Design review of the part built by this model. Coordinates are the model's own, in mm. A direction names the side the tool comes from. Give positions to 0.01 mm unless a question says otherwise; leave off trailing zeros. Write each loop counter-clockwise with the first axis right and the second up, starting at its lowest first coordinate (ties: lowest second). Pieces come first, ordered by that corner, then holes. Notation, with made-up numbers: M 24,74.5 L 33,74.5 A13 cw 33,83.5 Z; hole C 80.25,-3 d1. An arc over 180 degrees is marked long. Write each question's results on one line, items separated by ' | '. Start each with the question number.
Autodesk Fusion 360 part; units mm, degrees
sketch "Sketch1" plane through (0, 0, 0) normal (0, 0, 1) x (1, 0, 0)
  circle A0 centre (0, 0) radius 22.75
  circle A1 centre (0, 0) radius 24.25
  dimension "d1" = 45.5
  dimension "d2" = 48.5
extrude "Extrude1" add sketch "Sketch1" along normal blind 33
sketch "Sketch2" plane through (0, 0, 0) normal (0, 1, 0) x (1, 0, 0)
  line L0 (-24.25, 0) -> (24.25, 0)
  line L1 (4.75, -6.25) -> (-4.75, -6.25)
  line L2 (-4.75, -6.25) -> (-4.75, -2.75)
  line L3 (-4.75, -2.75) -> (4.75, -2.75)
  line L4 (4.75, -2.75) -> (4.75, -6.25)
  line L5 (4.75, -6.25) -> (-4.75, -2.75) construction
  line L6 (-4.75, -6.25) -> (4.75, -2.75) construction
  point P0 (0, -4.5)
  dimension "d9" = 9.5
  dimension "d10" = 3.5
  dimension "d11" = 2.75
extrude "Extrude2" cut sketch "Sketch2" along normal mid plane 66
sketch "Sketch3" plane through (0, 0, 33) normal (0, 0, 1) x (-1, 0, 0)
  circle A0 centre (0, 0) radius 22.75
  circle A1 centre (0, 0) radius 24.25
  circle A2 centre (0, 0) radius 25
  circle A3 centre (0, 0) radius 22.75
extrude "Extrude3" add sketch "Sketch3" along normal blind 3 contours A1 | A2
sketch "Sketch4" plane through (0, 0, 36) normal (0, 0, 1) x (-1, 0, 0)
  circle A0 centre (0, 0) radius 22.75
  circle A1 centre (0, 0) radius 25
  circle A2 centre (0, 0) radius 23.25
  circle A3 centre (0, 0) radius 22
  dimension "d18" = 46.5
  dimension "d19" = 44
ref_plane "WorkPlane2" through (0, 0, 43) normal (0, 0, 1) x (-1, 0, 0)
sketch "Sketch6" plane through (0, 0, 43) normal (0, 0, 1) x (1, 0, 0)
  circle A0 centre (0, 0) radius 22
  circle A1 centre (0, 0) radius 23.25
  dimension "d26" = 44
  dimension "d27" = 46.5
extrude "Extrude4" add sketch "Sketch6" against normal blind 7
ref_plane "WorkPlane1" through (0, 0, 56) normal (0, 0, 1) x (-1, 0, 0)
sketch "Sketch5" plane through (0, 0, 56) normal (0, 0, 1) x (1, 0, 0)
  circle A0 centre (0, 0) radius 22.75
  circle A1 centre (0, 0) radius 21.25
  dimension "d21" = 45.5
  dimension "d22" = 42.5
loft "Loft1" add profiles "Sketch6", "Sketch5" section 1 section 2
loft "Loft2" cut profiles "Sketch5", "Sketch6" section 1 contours A1 section 2 contours A0
chamfer "Chamfer1" distance 1.75 angle 45 1 edges at (-21.6766, 8.4076, 36)
chamfer "Chamfer3" distance 0.75 angle 45 1 edges at (21.2104, -8.2268, 36)
chamfer "Chamfer4" distance 0.75 angle 45 1 edges at (-22.6089, -8.7692, 33)
fillet "Fillet1" radius 1.75 8 edges at (-4.75, -23.0144, 6.25) (-4.75, -23.0144, 2.75) (4.75, -23.0144, 6.25) (4.75, -23.0144, 2.75) (4.75, 23.0144, 2.75) (4.75, 23.0144, 6.25) (-4.75, 23.0144, 6.25) (-4.75, 23.0144, 2.75)
Q1. The part is to be moulded in two halves that separate along Y. For faces 4 (the flat face through (-19, 10, 56)), 5 (the cylindrical face through (-4.769, -21.477, 39.549)), 6 (the cylindrical face through (22.176, 6.984, 40.412)), say which applies: pulls with the +Y half, pulls with the -Y half, needs draft (parallel to the pull), parting line crosses it, or undercut.
Q2. Wall thickness on line 1 along Y through (x, z) = (0, 18); line 2 along Y through (x, z) = (3, 21); line 3 along X through (y, z) = (18.5, 45): over which ranges is each line inside the solid? List them lowest first. Write a range as from..to.
Q3. For faces 1 (the conical face through (-5.064, 22.804, 37.64)), 2 (the cylindrical face through (4.251, -23.143, 3.276)), 3 (the cylindrical face through (11.19, 21.514, 15.899)), list the 3-axis set-ups (+Z, -Z, +X, -X, +Y, -Y) from which the entire face can be reached by the end or side of a thin tool; tool diameter is ignored.
Q4. For pin 1 Ø8 at (x, z) = (-14.5, 50) entering from -Y; pin 2 Ø12 at (x, z) = (6.5, 14.5) entering from -Y; pin 3 Ø3 at (y, z) = (4.5, 34) entering from -X; pin 4 Ø25 at (x, y) = (-1, -0.5) entering from -Z, all flat-tipped, find the tip position at first contact; note any pin that passes through.
Q5. We need section B-B on z = 24. Write out the cut boundary in (x, y).
Answer sheet:
1) face 4: needs draft | face 5: undercut | face 6: parting line crosses it
2) line 1: -24.25..-22.75, 22.75..24.25 | line 2: -24.06..-22.55, 22.55..24.06 | line 3: -13.95..-11.69, 11.69..13.95
3) face 1: +Z | face 2: +Y, -Y | face 3: -Z
4) pin 1: y = -20.45 | pin 2: y = -24.24 | pin 3: x = -24.82 | pin 4: through
5) outline: C 0,0 d48.5; hole C 0,0 d45.5
